from build123d import *

# Parameters (mm, degrees)
SKETCH1_W           = 50.8
SKETCH1_H           = 25.4
SKETCH1_W_2         = 47.625
SKETCH1_H_2         = 22.225
BOSS_EXTRUDE1_DEPTH = 127
SKETCH3_R           = 2.5527
CUT_EXTRUDE1_DEPTH  = 1.5875
SKETCH5_R           = 4.7625
SKETCH5_R_2         = 2.5527
CUT_EXTRUDE2_DEPTH  = 1.5875
SKETCH6_R           = 2.4892
CUT_EXTRUDE3_DEPTH  = 138.371503595
SKETCH11_R          = 9.906
SKETCH11_R_2        = 2.5527
SKETCH11_R_3        = 1.4224
CUT_EXTRUDE4_DEPTH  = 132.982271537


with BuildPart() as part:
    # Sketch1 → Boss-Extrude1 (new, symmetric)
    with BuildSketch(Plane.XY):
        Rectangle(SKETCH1_W, SKETCH1_H)
        Rectangle(SKETCH1_W_2, SKETCH1_H_2, mode=Mode.SUBTRACT)
    extrude(amount=BOSS_EXTRUDE1_DEPTH, both=True)

    # Sketch3 → Cut-Extrude1 (cut)
    with BuildSketch(Plane(origin=(0, 12.7, 0), x_dir=(1, 0, 0), z_dir=(0, 1, 0))):
        with Locations(Location((-12.7, -114.3, 0), (0, 0, 270))):
            Circle(SKETCH3_R)
        with Locations(Location((0, -114.3, 0), (0, 0, 270))):
            Circle(SKETCH3_R)
        with Locations(Location((-12.7, 114.3, 0), (0, 0, 270))):
            Circle(SKETCH3_R)
        with Locations(Location((0, 114.3, 0), (0, 0, 270))):
            Circle(SKETCH3_R)
    extrude(amount=-CUT_EXTRUDE1_DEPTH, mode=Mode.SUBTRACT)

    # Sketch5 → Cut-Extrude2 (cut)
    with BuildSketch(Plane.XZ.offset(12.7)):
        with Locations(Location((0, -114.3, 0), (0, 0, 270))):
            Circle(SKETCH5_R)
        with Locations(Location((0, -114.3, 0), (0, 0, 90))):
            Circle(SKETCH5_R_2, mode=Mode.SUBTRACT)
        with Locations(Location((0, -114.3, 0), (0, 0, 90))):
            Circle(SKETCH5_R_2)
        with Locations(Location((-12.7, -114.3, 0), (0, 0, 270))):
            Circle(SKETCH5_R)
        with Locations(Location((-12.7, -114.3, 0), (0, 0, 90))):
            Circle(SKETCH5_R_2, mode=Mode.SUBTRACT)
        with Locations(Location((-12.7, -114.3, 0), (0, 0, 90))):
            Circle(SKETCH5_R_2)
        with Locations(Location((0, 114.3, 0), (0, 0, 270))):
            Circle(SKETCH5_R)
        with Locations(Location((0, 114.3, 0), (0, 0, 90))):
            Circle(SKETCH5_R_2, mode=Mode.SUBTRACT)
        with Locations(Location((0, 114.3, 0), (0, 0, 90))):
            Circle(SKETCH5_R_2)
        with Locations(Location((-12.7, 114.3, 0), (0, 0, 270))):
            Circle(SKETCH5_R)
        with Locations(Location((-12.7, 114.3, 0), (0, 0, 90))):
            Circle(SKETCH5_R_2, mode=Mode.SUBTRACT)
        with Locations(Location((-12.7, 114.3, 0), (0, 0, 90))):
            Circle(SKETCH5_R_2)
    extrude(amount=-CUT_EXTRUDE2_DEPTH, mode=Mode.SUBTRACT)

    # Sketch6 → Cut-Extrude3 (cut, through all)
    with BuildSketch(Plane(origin=(25.4, 0, 0), x_dir=(0, 0, -1), z_dir=(1, 0, 0))):
        with Locations((-114.3, -3.175)):
            Circle(SKETCH6_R)
        with Locations((114.3, -3.175)):
            Circle(SKETCH6_R)
        with Locations((-102.87, -3.175)):
            Circle(SKETCH6_R)
        with Locations((-80.01, -3.175)):
            Circle(SKETCH6_R)
        with Locations((-57.15, -3.175)):
            Circle(SKETCH6_R)
        with Locations((-34.29, -3.175)):
            Circle(SKETCH6_R)
        with Locations((-11.43, -3.175)):
            Circle(SKETCH6_R)
        with Locations((11.43, -3.175)):
            Circle(SKETCH6_R)
        with Locations((34.29, -3.175)):
            Circle(SKETCH6_R)
        with Locations((57.15, -3.175)):
            Circle(SKETCH6_R)
        with Locations((80.01, -3.175)):
            Circle(SKETCH6_R)
        with Locations((102.87, -3.175)):
            Circle(SKETCH6_R)
    extrude(amount=-CUT_EXTRUDE3_DEPTH, mode=Mode.SUBTRACT)

    # Sketch11 → Cut-Extrude4 (cut, through all)
    with BuildSketch(Plane(origin=(0, 12.7, 0), x_dir=(1, 0, 0), z_dir=(0, 1, 0))):
        with Locations(Location((0, -22.225, 0), (0, 0, 270))):
            Circle(SKETCH11_R)
        with Locations(Location((0, 3.175, 0), (0, 0, 270))):
            Circle(SKETCH11_R_2)
        with Locations(Location((0, -47.625, 0), (0, 0, 270))):
            Circle(SKETCH11_R_2)
        with Locations(Location((-15.875, 19.05, 0), (0, 0, 270))):
            Circle(SKETCH11_R_2)
        with Locations(Location((-15.875, 38.1, 0), (0, 0, 270))):
            Circle(SKETCH11_R_2)
        with Locations(Location((-3.175, 19.05, 0), (0, 0, 270))):
            Circle(SKETCH11_R_2)
        with Locations(Location((-3.175, 38.1, 0), (0, 0, 270))):
            Circle(SKETCH11_R_2)
        with Locations(Location((-17.78, -4.085771792, 0), (0, 0, 270))):
            Circle(SKETCH11_R_2)
        with Locations(Location((17.78, -40.364228208, 0), (0, 0, 270))):
            Circle(SKETCH11_R_2)
        with Locations(Location((-9.525, 73.66, 0), (0, 0, 270))):
            Circle(SKETCH11_R_3)
        with Locations(Location((-1.524999998, 73.66, 0), (0, 0, 270))):
            Circle(SKETCH11_R_3)
    extrude(amount=-CUT_EXTRUDE4_DEPTH, mode=Mode.SUBTRACT)


solid = part.part
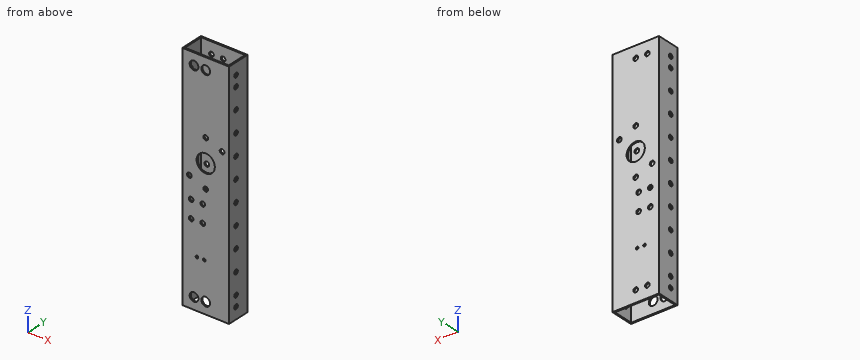
Work out the finished part from the listing and answer in its coordinate system (mm). Round coordinates to 2 decimals unless told otherwise and drop trailing zeros. Write each loop counter-clockwise with the first axis right and the second up, starting at its lowest first coordinate (ties: lowest second). Pieces come first, ordered by that corner, then holes.
1) Given pin 1 Ø4.5 at (x, z) = (-12.7, 114.3) entering from +Y; pin 2 Ø5.5 at (x, z) = (-12.7, -114.3) entering from -Y, each flat-ended and moving along its own axis, determine where each tip first touches the part or whether it passes through.
2) Straight lines are drawn through the part: line 1 (X direction, y = -11.85, z = 114.3); line 2 (X direction, y = -12.2, z = -38.1); line 3 (Y direction, x = 11.5, z = 99). For each, find the intervals that lie inside material, in ascending order.
3) A cutting plane is placed at C-C (z = -114.3). Give the number of separate pieces and of enclosed holes in the cut face, plus the area to 3 significant figures.
4) A cutting plane is placed at B-B (y = 2.25). Give the vertices of the cut face in (x, z), plus the area to 3 significant figures.
5) A cutting plane is placed at A-A (z = -19.05). Give the vertices of the cut face in (x, y), plus the area to 3 significant figures.
6) A cutting plane is placed at D-D (z = 65). Give the vertices of the cut face in (x, y), plus the area to 3 significant figures.
Completed:
1. pin 1: passes through
1. pin 2: stops at y = 11.11
2. line 1: x = -25.4 to -17.46, -7.94 to -4.76, 4.76 to 25.4
2. line 2: x = -25.4 to -18.43, -13.32 to -5.73, -0.62 to 25.4
2. line 3: y = -12.7 to -11.11, 11.11 to 12.7
3. separate pieces: 6
3. enclosed holes: 0
3. area: 170 mm2
4. outline: (-25.4, -127) - (-23.81, -127) - (-23.81, 127) - (-25.4, 127) - close; (23.81, -127) - (25.4, -127) - (25.4, 127) - (23.81, 127) - close
4. area: 806 mm2
5. outline: (-25.4, -12.7) - (-18.43, -12.7) - (-18.43, -11.11) - (-23.81, -11.11) - (-23.81, 11.11) - (-18.43, 11.11) - (-18.43, 12.7) - (-25.4, 12.7) - close; (-13.32, -12.7) - (-5.73, -12.7) - (-5.73, -11.11) - (-13.32, -11.11) - close; (-13.32, 11.11) - (-5.73, 11.11) - (-5.73, 12.7) - (-13.32, 12.7) - close; (-0.62, -12.7) - (25.4, -12.7) - (25.4, 12.7) - (-0.62, 12.7) - (-0.62, 11.11) - (23.81, 11.11) - (23.81, -11.11) - (-0.62, -11.11) - close
5. area: 199 mm2
6. outline: (-25.4, -12.7) - (25.4, -12.7) - (25.4, 12.7) - (-25.4, 12.7) - close; hole (-23.81, -11.11) - (23.81, -11.11) - (23.81, 11.11) - (-23.81, 11.11) - close
6. area: 232 mm2
